Can you work these out from the model? Positions are in its coordinate system, mm. Face numbers are marked on the shaded views. A direction names the side the tool comes from. Coordinates: 2 decimals unless noted, no trailing zeros. Write each loop counter-clockwise with the first axis right and the second up, starting at its lowest first coordinate (ties: lowest second). Pieces come first, ordered by that corner, then holes. Notation, with made-up numbers: (27.5, 22) - (36.5, 22) arc R16 ccw to (36.5, 47) - close; hole circle Ø1 at (75.25, 4). An arc over 180 degrees is marked (long way). Use one line per item in the form item = value. Start each with the question number.
(1) If we section it at A-A on x = 60: Please give me the cut outline in (y, z).
(2) On a 3-axis mill with a long thin cutter (end or side, diameter ignored), from which of +Z, -Z, +X, -X, +Y, -Y can I reach the whole of each face in a straight line? I mean the marked faces 1 and 2. Say none if no direction works.
(3) If we section it at C-C on y = -22: Please give me the cut outline in (x, z), then the cut area to 3 significant figures.
(4) If we section it at B-B on y = 25: Please give me the cut outline in (x, z).
(5) If we section it at D-D on x = -14.5: Please give me the cut outline in (y, z), then the cut area to 3 significant figures.
(6) Thinking about a two-plate mould opening in X: for the marked faces 3, 4 and 5, which applies, pulls with the +X half, pulls with the -X half, needs draft (parallel to the pull), parting line crosses it, or undercut?
(7) If I drill on probe 1 along X at (y, z) = (36.5, 9.5); probe 2 along Y at (x, z) = (-60, 8.75); probe 3 along Z at (x, y) = (-144, 0.5), over which ranges is the centre line in solid material (lowest first)? Write a range as from..to.
(8) For pin 1 Ø10 at (x, z) = (102.5, 5) entering from +Y; pin 2 Ø7 at (x, y) = (-60, -22) entering from -Z; pin 3 Ø1.5 at (x, z) = (103, 6.5) entering from -Y, each with a flat end and sliding along its axis, tell me the tip position at first contact or that it passes through.
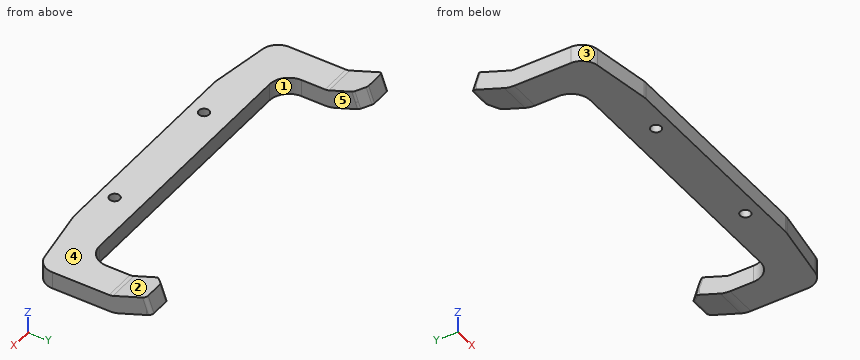
```python
from build123d import *

# Parameters (mm, degrees)
SKETCH1_R              = 4.5
EXTRUDE1_DEPTH         = 15
PROCESS_BENDS1_START   = -159
PROCESS_BENDS1_DEPTH   = 318
PROCESS_BENDS1_2_DEPTH = 28
PROCESS_BENDS1_START_2 = 131
PROCESS_BENDS1_3_DEPTH = 28
PROCESS_BENDS1_START_3 = -0.699454706
PROCESS_BENDS1_4_DEPTH = 14.999999999
PROCESS_BENDS1_START_4 = 7.710911858
PROCESS_BENDS1_5_DEPTH = 6.589633435


with BuildPart() as part:
    # Sketch1 → Extrude1 (new body)
    with BuildSketch(Plane.XY):
        with BuildLine():
            Line((-114, 0), (114, 0))
            ThreePointArc((114, 0), (126.02081528, 4.97918472), (131, 17))
            Line((131, 17), (131, 63.757359313))
            ThreePointArc((131, 63.757359313), (131.228361402, 64.90540961), (131.878679656, 65.878679656))
            Line((131.878679656, 65.878679656), (138.121320344, 72.121320344))
            ThreePointArc((138.121320344, 72.121320344), (139.09459039, 72.771638598), (140.242640687, 73))
            Line((140.242640687, 73), (156, 73))
            ThreePointArc((156, 73), (158.121320344, 72.121320344), (159, 70))
            Line((159, 70), (159, -12.052185537))
            ThreePointArc((159, -12.052185537), (155.406089484, -21.793906262), (146.346516976, -26.867510646))
            Line((146.346516976, -26.867510646), (96.165991373, -34.815325109))
            ThreePointArc((96.165991373, -34.815325109), (94.996360834, -34.953760006), (93.819474398, -35))
            Line((93.819474398, -35), (-93.819474398, -35))
            ThreePointArc((-93.819474398, -35), (-94.996360834, -34.953760006), (-96.165991373, -34.815325109))
            Line((-96.165991373, -34.815325109), (-146.346516976, -26.867510646))
            ThreePointArc((-146.346516976, -26.867510646), (-155.406089484, -21.793906262), (-159, -12.052185537))
            Line((-159, -12.052185537), (-159, 70))
            ThreePointArc((-159, 70), (-158.121320344, 72.121320344), (-156, 73))
            Line((-156, 73), (-140.242640687, 73))
            ThreePointArc((-140.242640687, 73), (-139.09459039, 72.771638598), (-138.121320344, 72.121320344))
            Line((-138.121320344, 72.121320344), (-131.878679656, 65.878679656))
            ThreePointArc((-131.878679656, 65.878679656), (-131.228361402, 64.90540961), (-131, 63.757359313))
            Line((-131, 63.757359313), (-131, 17))
            ThreePointArc((-131, 17), (-126.02081528, 4.97918472), (-114, 0))
        make_face()
        with Locations((60, -22)):
            Circle(SKETCH1_R, mode=Mode.SUBTRACT)
        with Locations(Location((-60, -22, 0), (0, 0, 180))):
            Circle(SKETCH1_R, mode=Mode.SUBTRACT)
    extrude(amount=EXTRUDE1_DEPTH)

    # Process-Bends1: read off the stored shape, not the designer's step
    # Process-Bends1 outline → Process-Bends1 (cut)
    with BuildSketch(Plane.YZ.offset(PROCESS_BENDS1_START)):
        with BuildLine():
            Line((73, 0), (73, 11.351504666))
            Line((73, 11.351504666), (45.954326321, 1.50768448))
            ThreePointArc((45.954326321, 1.50768448), (41.745027179, 0.379806175), (37.403822738, 0))
            Line((37.403822738, 0), (73, 0))
        make_face()
    extrude(amount=PROCESS_BENDS1_DEPTH, mode=Mode.SUBTRACT)

    # Process-Bends1 2 outline → Process-Bends1 2 (add)
    with BuildSketch(Plane.YZ.offset(PROCESS_BENDS1_START)):
        with BuildLine():
            Line((74.524574191, 11.906404291), (69.394272041, 26.001793603))
            Line((69.394272041, 26.001793603), (40.824024171, 15.603073792))
            ThreePointArc((40.824024171, 15.603073792), (39.140304514, 15.15192247), (37.403822738, 15))
            Line((37.403822738, 15), (73, 15))
            Line((73, 15), (73, 11.351504666))
            Line((73, 11.351504666), (74.524574191, 11.906404291))
        make_face()
    extrude(amount=PROCESS_BENDS1_2_DEPTH)

    # Process-Bends1 3 outline → Process-Bends1 3 (add)
    with BuildSketch(Plane.YZ.offset(PROCESS_BENDS1_START_2)):
        with BuildLine():
            Line((74.524574191, 11.906404291), (69.394272041, 26.001793603))
            Line((69.394272041, 26.001793603), (40.824024171, 15.603073792))
            ThreePointArc((40.824024171, 15.603073792), (39.140304514, 15.15192247), (37.403822738, 15))
            Line((37.403822738, 15), (73, 15))
            Line((73, 15), (73, 11.351504666))
            Line((73, 11.351504666), (74.524574191, 11.906404291))
        make_face()
    extrude(amount=PROCESS_BENDS1_3_DEPTH)

    # Process-Bends1 4 outline → Process-Bends1 4 (cut)
    with BuildSketch(Plane(origin=(0, 0, 0), x_dir=(1, 0, 0), z_dir=(0, 0.34202014332567, -0.939692620785908)).offset(PROCESS_BENDS1_START_3)):
        with BuildLine():
            ThreePointArc((140.242640687, -74.102422537), (139.09459039, -73.874061134), (138.121320344, -73.22374288))
            Line((138.121320344, -73.22374288), (131.878679656, -66.981102193))
            ThreePointArc((131.878679656, -66.981102193), (131.228361402, -66.007832146), (131, -64.859781849))
            Line((131, -64.859781849), (131, -74.102422537))
            Line((131, -74.102422537), (140.242640687, -74.102422537))
        make_face()
        with BuildLine():
            ThreePointArc((159, -71.102422537), (158.121320344, -73.22374288), (156, -74.102422537))
            Line((156, -74.102422537), (159, -74.102422537))
            Line((159, -74.102422537), (160, -74.102422548))
            Line((160, -74.102422548), (160, -61))
            Line((160, -61), (159.000000001, -61))
            Line((159.000000001, -61), (159, -71.102422537))
        make_face()
        with BuildLine():
            Line((-140.242640687, -74.102422537), (-131, -74.102422537))
            Line((-131, -74.102422537), (-131, -64.859781849))
            ThreePointArc((-131, -64.859781849), (-131.228361402, -66.007832146), (-131.878679656, -66.981102193))
            Line((-131.878679656, -66.981102193), (-138.121320344, -73.22374288))
            ThreePointArc((-138.121320344, -73.22374288), (-139.09459039, -73.874061134), (-140.242640687, -74.102422537))
        make_face()
        with BuildLine():
            Line((-159, -74.102422537), (-156, -74.102422537))
            ThreePointArc((-156, -74.102422537), (-158.121320344, -73.22374288), (-159, -71.102422537))
            Line((-159, -71.102422537), (-159.000000001, -61))
            Line((-159.000000001, -61), (-160, -61))
            Line((-160, -61), (-160, -74.102422548))
            Line((-160, -74.102422548), (-159, -74.102422537))
        make_face()
    extrude(amount=PROCESS_BENDS1_4_DEPTH, mode=Mode.SUBTRACT)

    # Process-Bends1 5 outline → Process-Bends1 5 (add)
    with BuildSketch(Plane(origin=(0, 0, 0), x_dir=(1, 0, 0), z_dir=(0, 0.34202014332567, -0.939692620785908)).offset(PROCESS_BENDS1_START_4)):
        with BuildLine():
            Line((131.878679656, -66.981102193), (138.121320344, -73.22374288))
            ThreePointArc((138.121320344, -73.22374288), (139.09459039, -73.874061134), (140.242640687, -74.102422537))
            Line((140.242640687, -74.102422537), (156, -74.102422537))
            ThreePointArc((156, -74.102422537), (158.121320344, -73.22374288), (159, -71.102422537))
            Line((159, -71.102422537), (159.000000001, -61))
            Line((159.000000001, -61), (131.000000004, -61))
            Line((131.000000004, -61), (131, -64.859781849))
            ThreePointArc((131, -64.859781849), (131.228361402, -66.007832146), (131.878679656, -66.981102193))
        make_face()
        with BuildLine():
            ThreePointArc((-131.878679656, -66.981102193), (-131.228361402, -66.007832146), (-131, -64.859781849))
            Line((-131, -64.859781849), (-131, -61))
            Line((-131, -61), (-159.000000001, -61))
            Line((-159.000000001, -61), (-159, -71.102422537))
            ThreePointArc((-159, -71.102422537), (-158.121320344, -73.22374288), (-156, -74.102422537))
            Line((-156, -74.102422537), (-140.242640687, -74.102422537))
            ThreePointArc((-140.242640687, -74.102422537), (-139.09459039, -73.874061134), (-138.121320344, -73.22374288))
            Line((-138.121320344, -73.22374288), (-131.878679656, -66.981102193))
        make_face()
    extrude(amount=PROCESS_BENDS1_5_DEPTH)


solid = part.part
```
Reported:
q1.outline = (-35, 0) - (-26.5, 0) - (-26.5, 15) - (-35, 15) - close; (-17.5, 0) - (0, 0) - (0, 15) - (-17.5, 15) - close
q2.face_1 = +Z, -Z, +Y
q2.face_2 = +Z, +X, -X, -Y
q3.outline = (-155.23, 0) - (-64.5, 0) - (-64.5, 15) - (-155.23, 15) - close; (-55.5, 0) - (55.5, 0) - (55.5, 15) - (-55.5, 15) - close; (64.5, 0) - (155.23, 0) - (155.23, 15) - (64.5, 15) - close
q3.area = 4,390 mm2
q4.outline = (-159, 0) - (-131, 0) - (-131, 15) - (-159, 15) - close; (131, 0) - (159, 0) - (159, 15) - (131, 15) - close
q5.outline = (-35, 0) - (0, 0) - (0, 15) - (-35, 15) - close
q5.area = 525 mm2
q6.face_3 = pulls with the -X half
q6.face_4 = needs draft
q6.face_5 = undercut
q7.probe_1 = -159..-131, 131..159
q7.probe_2 = -35..-26.5, -17.5..0
q7.probe_3 = 0..15
q8.pin_1 = 0
q8.pin_2 = through
q8.pin_3 = -33.85
